Part model, mm, in its own coordinate system. Face numbers are marked on the shaded views. A direction names the side the tool comes from. Round coordinates to 2 decimals unless told otherwise and drop trailing zeros. Loops run counter-clockwise (first coordinate to the right, second up) from the corner with the lowest first, then second, coordinate; pieces in that order, holes last. Notation, with made-up numbers: (36.25, 14.25) - (78.25, 14.25) arc R20 ccw to (78.25, 52.25) - close; hole circle Ø1 at (19, 72.25). An arc over 180 degrees is marked (long way). Put each result on its own line as item: value.
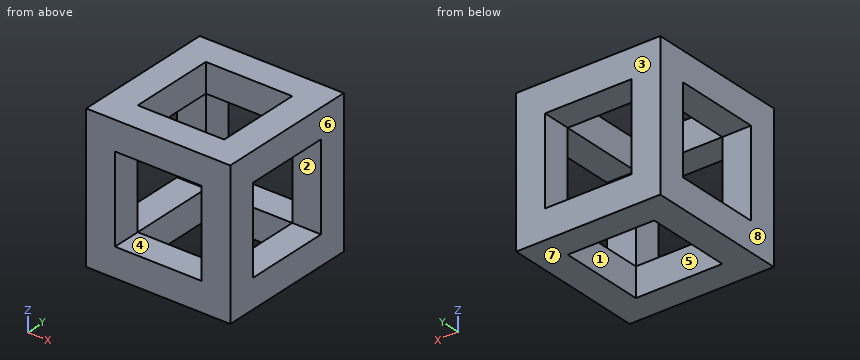
from build123d import *

# Parameters (mm, degrees)
F0_W     = 20
F0_H     = 20
F1_DEPTH = 20
F2_W     = 12
F2_H     = 12
F3_DEPTH = 90
F4_W     = 12
F4_H     = 12
F5_DEPTH = 60.3
F6_W     = 12
F6_H     = 12
F7_DEPTH = 36


with BuildPart() as f1:
    # F0 (on Top) → F1 (new body)
    with BuildSketch(Plane.XY):
        with Locations((-41.299911, -23.300817)):
            Rectangle(F0_W, F0_H)
    extrude(amount=F1_DEPTH)

    # F2 (on Right) → F3 (cut)
    with BuildSketch(Plane.YZ):
        with Locations((-23.300817, 10)):
            Rectangle(F2_W, F2_H)
    extrude(amount=-F3_DEPTH, mode=Mode.SUBTRACT)

    # F4 (on Front) → F5 (cut)
    with BuildSketch(Plane.XZ):
        with Locations((-41.299911, 10)):
            Rectangle(F4_W, F4_H)
    extrude(amount=F5_DEPTH, mode=Mode.SUBTRACT)

    # F6 (on Top) → F7 (cut)
    with BuildSketch(Plane.XY):
        with Locations((-41.299911, -23.300817)):
            Rectangle(F6_W, F6_H)
    extrude(amount=F7_DEPTH, mode=Mode.SUBTRACT)


solid = f1.part
1. Pin check, flat tip, straight feed: P1, Ø4.5, axis at x = -42.5, y = -15, coming from the -Z side. Stop position of the tip, or through.
A:
P1: stops at z = 0
2. Tool access for the marked faces 1, 2, 3 and 4: list every direction of +Z, -Z, +X, -X, +Y, -Y with a clear straight run to the whole face (end or side of a thin tool).
A:
face 1: +Z, -Z
face 2: +X, -X
face 3: +Z, -Z, +X, -X, +Y
face 4: +Y, -Y
3. Band-saw the part on D-D (z = 3). List the corners of the cut face in (x, y), plus the area to 3 significant figures.
A:
outline: (-51.3, -33.3) - (-31.3, -33.3) - (-31.3, -13.3) - (-51.3, -13.3) - close; hole (-47.3, -29.3) - (-35.3, -29.3) - (-35.3, -17.3) - (-47.3, -17.3) - close
area: 256 mm²
4. Band-saw the part on A-A (y = -23.75). List the corners of the cut face in (x, z).
A:
outline: (-51.3, 0) - (-47.3, 0) - (-47.3, 4) - (-51.3, 4) - close; (-51.3, 16) - (-47.3, 16) - (-47.3, 20) - (-51.3, 20) - close; (-35.3, 0) - (-31.3, 0) - (-31.3, 4) - (-35.3, 4) - close; (-35.3, 16) - (-31.3, 16) - (-31.3, 20) - (-35.3, 20) - close
5. Probe line 1 along X through (y, z) = (-17, 9.75); line 2 along Z through (x, y) = (-38, -14.25); line 3 along Y through (x, z) = (-49.25, 11.75). List the from-to ranges inside material, lowest first. Write a range as [from, to].
A:
line 1: x = [-51.3, -47.3], [-35.3, -31.3]
line 2: z = [0, 4], [16, 20]
line 3: y = [-33.3, -29.3], [-17.3, -13.3]
6. Band-saw the part on C-C (y = -30). List the corners of the cut face in (x, z).
A:
outline: (-51.3, 0) - (-31.3, 0) - (-31.3, 20) - (-51.3, 20) - close; hole (-47.3, 4) - (-35.3, 4) - (-35.3, 16) - (-47.3, 16) - close
7. Band-saw the part on B-B (z = 11.5). List the corners of the cut face in (x, y).
A:
outline: (-51.3, -33.3) - (-47.3, -33.3) - (-47.3, -29.3) - (-51.3, -29.3) - close; (-51.3, -17.3) - (-47.3, -17.3) - (-47.3, -13.3) - (-51.3, -13.3) - close; (-35.3, -33.3) - (-31.3, -33.3) - (-31.3, -29.3) - (-35.3, -29.3) - close; (-35.3, -17.3) - (-31.3, -17.3) - (-31.3, -13.3) - (-35.3, -13.3) - close
8. Two-plate mould, pull along X, no slides. Class the marked faces 5, 6, 7 and 8: pulls with the +X half, pulls with the -X half, needs draft (parallel to the pull), parting line crosses it, or undercut.
A:
face 5: undercut
face 6: pulls with the +X half
face 7: needs draft
face 8: pulls with the -X half
